Design review of the part built by this model. Coordinates are the model's own, in mm. A direction names the side the tool comes from. Give positions to 0.01 mm unless a question says otherwise; leave off trailing zeros. Write each loop counter-clockwise with the first axis right and the second up, starting at its lowest first coordinate (ties: lowest second). Pieces come first, ordered by that corner, then holes. Notation, with made-up numbers: (-22, -27.5) -> (12, -27.5) arc R24 cw to (12, -9.5) -> close; hole circle Ø4 at (89.5, 53.5). An arc over 180 degrees is marked (long way). Answer as a JSON object with one key per item and string values.
```python
from build123d import *
from build123d.topology import SkipClean

# Parameters (mm, degrees)
ESQUISSE2_R             = 53
ESQUISSE2_R_2           = 3
BOSS_EXTRU_1_DEPTH      = 10
ESQUISSE3_R             = 22
ESQUISSE3_R_2           = 3
BOSS_EXTRU_2_DEPTH      = 20
ENL_V_MAT_EXTRU_1_DEPTH = 6
ENL_V_MAT_EXTRU_2_DEPTH = 81.734131568
ESQUISSE7_R             = 2
ENL_V_MAT_EXTRU_3_DEPTH = 81.734131568


with BuildPart() as part:
    # Esquisse2 → Boss.-Extru.1 (new body)
    with BuildSketch(Plane.XY):
        Circle(ESQUISSE2_R)
        with Locations((0, -15)):
            Circle(ESQUISSE2_R_2, mode=Mode.SUBTRACT)
        with Locations((12.990381057, -7.5)):
            Circle(ESQUISSE2_R_2, mode=Mode.SUBTRACT)
        with Locations((12.990381057, 7.5)):
            Circle(ESQUISSE2_R_2, mode=Mode.SUBTRACT)
        with Locations((0, 15)):
            Circle(ESQUISSE2_R_2, mode=Mode.SUBTRACT)
        with Locations((-12.990381057, 7.5)):
            Circle(ESQUISSE2_R_2, mode=Mode.SUBTRACT)
        with BuildLine():
            Line((-26.649284405, 31.157914575), (-16.836249468, 14.161239488))
            ThreePointArc((-16.836249468, 14.161239488), (-21.250368178, 5.694018992), (-21.661239488, -3.845868412))
            Line((-21.661239488, -3.845868412), (-38.657914575, -13.658903349))
            ThreePointArc((-38.657914575, -13.658903349), (-39.602958878, 10.611580849), (-26.649284405, 31.157914575))
        make_face(mode=Mode.SUBTRACT)
        with BuildLine():
            Line((-13.658903349, 38.657914575), (-3.845868412, 21.661239488))
            ThreePointArc((-3.845868412, 21.661239488), (5.694018992, 21.250368178), (14.161239488, 16.836249468))
            Line((14.161239488, 16.836249468), (31.157914575, 26.649284405))
            ThreePointArc((31.157914575, 26.649284405), (10.611580849, 39.602958878), (-13.658903349, 38.657914575))
        make_face(mode=Mode.SUBTRACT)
        with BuildLine():
            Line((38.657914575, 13.658903349), (21.661239488, 3.845868412))
            ThreePointArc((21.661239488, 3.845868412), (21.250368178, -5.694018992), (16.836249468, -14.161239488))
            Line((16.836249468, -14.161239488), (26.649284405, -31.157914575))
            ThreePointArc((26.649284405, -31.157914575), (39.602958878, -10.611580849), (38.657914575, 13.658903349))
        make_face(mode=Mode.SUBTRACT)
        with BuildLine():
            Line((13.658903349, -38.657914575), (3.845868412, -21.661239488))
            ThreePointArc((3.845868412, -21.661239488), (-5.694018992, -21.250368178), (-14.161239488, -16.836249468))
            Line((-14.161239488, -16.836249468), (-31.157914575, -26.649284405))
            ThreePointArc((-31.157914575, -26.649284405), (-10.611580849, -39.602958878), (13.658903349, -38.657914575))
        make_face(mode=Mode.SUBTRACT)
    extrude(amount=BOSS_EXTRU_1_DEPTH)

    # Esquisse3 → Boss.-Extru.2 (add)
    with BuildSketch(Plane.XY.offset(10)):
        with Locations(Location((0, 0, 0), (0, 0, 190.067729528))):
            Circle(ESQUISSE3_R)
        with Locations((-12.990381057, 7.5)):
            Circle(ESQUISSE3_R_2, mode=Mode.SUBTRACT)
        with Locations((0, 15)):
            Circle(ESQUISSE3_R_2, mode=Mode.SUBTRACT)
        with Locations((12.990381057, 7.5)):
            Circle(ESQUISSE3_R_2, mode=Mode.SUBTRACT)
        with Locations((12.990381057, -7.5)):
            Circle(ESQUISSE3_R_2, mode=Mode.SUBTRACT)
        with Locations((0, -15)):
            Circle(ESQUISSE3_R_2, mode=Mode.SUBTRACT)
    extrude(amount=BOSS_EXTRU_2_DEPTH)

    # Esquisse4 → Enlèv. mat.-Extru.1 (cut)
    with BuildSketch(Plane(origin=(0, 0, 0), x_dir=(-1, 0, 0), z_dir=(0, 0, -1))):
        Polygon((15.877132403, 2.5), (18.763883749, 7.5), (15.877132403, 12.5), (10.103629711, 12.5), (7.216878365, 7.5), (10.103629711, 2.5), align=None)
        Polygon((-2.886751346, 20), (-5.773502692, 15), (-2.886751346, 10), (2.886751346, 10), (5.773502692, 15), (2.886751346, 20), align=None)
        Polygon((-18.763883749, 7.5), (-15.877132403, 2.5), (-10.103629711, 2.5), (-7.216878365, 7.5), (-10.103629711, 12.5), (-15.877132403, 12.5), align=None)
        Polygon((-15.877132403, -12.5), (-10.103629711, -12.5), (-7.216878365, -7.5), (-10.103629711, -2.5), (-15.877132403, -2.5), (-18.763883749, -7.5), align=None)
        Polygon((2.886751346, -20), (5.773502692, -15), (2.886751346, -10), (-2.886751346, -10), (-5.773502692, -15), (-2.886751346, -20), align=None)
    extrude(amount=-ENL_V_MAT_EXTRU_1_DEPTH, mode=Mode.SUBTRACT)

    # Esquisse5 → Enlèv. mat.-Extru.2 (cut, through all)
    with SkipClean():  # the faces are left unmerged after this step: merging them gives an invalid solid
        with BuildSketch(Plane(origin=(0, 0, 0), x_dir=(-1, 0, 0), z_dir=(0, 0, -1))):
            with BuildLine():
                Line((2.384210575, -21.870426149), (20.132449924, 8.870426149))
                Line((20.132449924, 8.870426149), (38.657914575, -13.658903349))
                ThreePointArc((38.657914575, -13.658903349), (35.507041555, -20.5), (31.157914575, -26.649284405))
                Line((31.157914575, -26.649284405), (2.384210575, -21.870426149))
            make_face()
        extrude(amount=-ENL_V_MAT_EXTRU_2_DEPTH, mode=Mode.SUBTRACT)

    # Esquisse7 → Enlèv. mat.-Extru.3 (cut, through all)
    with SkipClean():  # the faces are left unmerged after this step: merging them gives an invalid solid
        with BuildSketch(Plane(origin=(0, 0, 0), x_dir=(-1, 0, 0), z_dir=(0, 0, -1))):
            with Locations((-43.301270189, 25)):
                Circle(ESQUISSE7_R)
            with Locations((25, 43.301270189)):
                Circle(ESQUISSE7_R)
            with Locations((43.301270189, -25)):
                Circle(ESQUISSE7_R)
            with Locations((-25, -43.301270189)):
                Circle(ESQUISSE7_R)
        extrude(amount=-ENL_V_MAT_EXTRU_3_DEPTH, mode=Mode.SUBTRACT)


solid = part.part
```
(1) Clearance check with flat-ended pins moving along their axes: pin 1 (5 mm diameter, centred on y = 16, z = 25.5, fed in from +X); pin 2 (6.5 mm diameter, centred on x = -13, z = 4, fed in from +Y); pin 3 (6 mm diameter, centred on y = -21.5, z = 3.5, fed in from +X). State where each tip first meets the part, or that it passes through.
Here are the results:
{"pin 1": "stops at x = 17.37", "pin 2": "stops at y = 52.1", "pin 3": "stops at x = 49.67"}
(2) We need section A-A, the plane z = 17. State the section outline as (x, y) points.
Here are the results:
{"outline": "(-20.13, 8.87) -> (-2.38, -21.87) arc R22 ccw (long way) to start; hole circle Ø6 at (-12.99, 7.5); hole circle Ø6 at (0, -15); hole circle Ø6 at (0, 15); hole circle Ø6 at (12.99, -7.5); hole circle Ø6 at (12.99, 7.5)"}
(3) We need section C-C, the plane x = 25. State the section outline as (y, z) points, then the cut area to 3 significant figures.
Here are the results:
{"outline": "(-46.73, 0) -> (-45.3, 0) -> (-45.3, 10) -> (-46.73, 10) -> close; (-41.3, 0) -> (-28.3, 0) -> (-28.3, 10) -> (-41.3, 10) -> close; (5.77, 0) -> (23.09, 0) -> (23.09, 10) -> (5.77, 10) -> close; (32.5, 0) -> (46.73, 0) -> (46.73, 10) -> (32.5, 10) -> close", "area": "460 mm²"}
(4) The part is to be moulded in two halves that separate along Y. For faces 4 (the flat face through (-1, 1, 0)), 5 (the flat face through (17.341, -9.965, 2.958)), say which applies: +Y half, -Y half, draft (parallel to the pull), parting line (faces both ways), or undercut.
Here are the results:
{"face 4": "draft", "face 5": "undercut"}
(5) For faces 1 (the flat face through (2, 0, 30)), 2 (the cylindrical face through (39.512, -10.945, 4.93)), 3 (the flat face through (17.341, 5.035, 2.958)), list the 3-axis set-ups (+Z, -Z, +X, -X, +Y, -Y) from which the entire face can be reached by the end or side of a thin tool; tool diameter is ignored.
Here are the results:
{"face 1": "+Z, +X, -X, +Y, -Y", "face 2": "+Z, -Z", "face 3": "-Z"}
(6) We need section D-D, the plane x = -25. State the section outline as (y, z) points.
Here are the results:
{"outline": "(-46.73, 0) -> (-32.5, 0) -> (-32.5, 10) -> (-46.73, 10) -> close; (28.3, 0) -> (41.3, 0) -> (41.3, 10) -> (28.3, 10) -> close; (45.3, 0) -> (46.73, 0) -> (46.73, 10) -> (45.3, 10) -> close"}
(7) We need section B-B, the plane y = 34. State the section outline as (x, z) points.
Here are the results:
{"outline": "(-40.66, 0) -> (-10.97, 0) -> (-10.97, 10) -> (-40.66, 10) -> close; (22.91, 0) -> (40.66, 0) -> (40.66, 10) -> (22.91, 10) -> close"}
(8) For line 1 along Y through (x, z) = (0, 16.25); line 2 along Y through (x, z) = (25, 8); line 3 along Y through (x, z) = (-12.5, 2.5), list the stretches that pass through material, from the lowest coordinate up.
Here are the results:
{"line 1": "y = -22 to -18, -12 to 12, 18 to 22", "line 2": "y = -46.73 to -45.3, -41.3 to -28.3, 5.77 to 23.09, 32.5 to 46.73", "line 3": "y = -51.5 to -39.05, -4.35 to 2.5, 12.5 to 36.65, 39.05 to 51.5"}
